Work out the finished part from the listing and answer in its coordinate system (mm). Face numbers are marked on the shaded views. Give positions to 0.01 mm unless a question says otherwise; leave off trailing zeros. Order: outer loops, then holes, each group sorted by start corner. A loop starts at its lowest first (then second) coordinate and runs counter-clockwise, first axis right, second up. Notation, with made-up numbers: M 36.25,50.5 L 42.25,50.5 A12 cw 42.25,64.5 Z; hole C 31,58 d1. An arc over 180 degrees is marked long. One line per item, written item: value.
from build123d import *

# Parameters (mm, degrees)
F1_DEPTH = 4
F2_R     = 1.99999
F3_R     = 1


# Not quite as in the source:
# - a fillet or chamfer is up to 0.001 mm smaller than in the source, because OpenCascade refuses the exact size


with BuildPart() as f1:
    # F0 (on Top) → F1 (new body)
    with BuildSketch(Plane.XY):
        Polygon((-28, 2), (-33, 2), (-33, -2), (-28, -2), (-28, -5), (-25, -5), (-25, -2), (25, -2), (25, -5), (28, -5), (28, -2), (33, -2), (33, 2), (28, 2), (28, 5), (25, 5), (25, 2), (-25, 2), (-25, 5), (-28, 5), align=None)
    extrude(amount=F1_DEPTH)

    # F2 (radius 2 in the source; OpenCascade refuses exactly that, so slightly less here)
    f2_edges = [f1.edges().sort_by_distance(p)[0] for p in [
        (33, -2, 2),
        (33, 2, 2),
        (-33, -2, 2),
        (-33, 2, 2),
    ]]
    fillet(f2_edges, radius=F2_R)

    # F3
    f3_edges = [f1.edges().sort_by_distance(p)[0] for p in [
        (-28, -5, 2),
        (-28, 5, 2),
        (28, -5, 2),
        (28, 5, 2),
        (-25, -5, 2),
        (-25, 5, 2),
        (25, 5, 2),
        (25, -5, 2),
        (25, -2, 2),
        (25, 2, 2),
        (-25, 2, 2),
        (-25, -2, 2),
    ]]
    fillet(f3_edges, radius=F3_R)


solid = f1.part
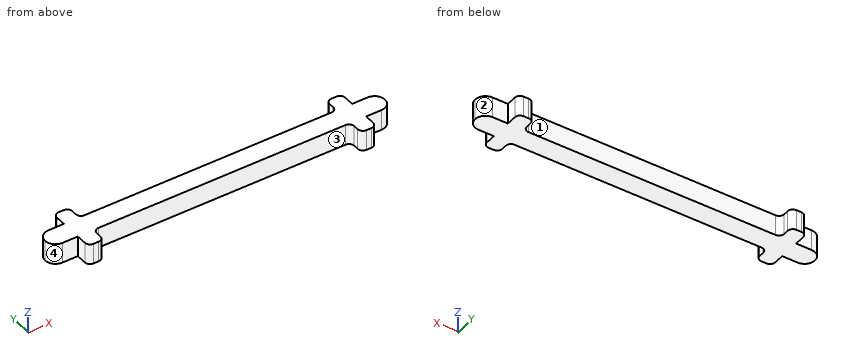
(1) Given P1, Ø0.6, axis at y = 3.5, z = 2.5, coming from the +X side; P2, Ø1.6, axis at y = -3, z = 2, coming from the -X side; P3, Ø2, axis at x = -10.5, z = 1.5, coming from the +Y side; P4, Ø6, axis at x = -6, y = 1, coming from the -Z side, each flat-ended and moving along its own axis, determine where each tip first touches the part or whether it passes through.
Findings:
P1: stops at x = 28
P2: stops at x = -28
P3: stops at y = 2
P4: stops at z = 0
(2) Determine the mould class of the marked faces 1, 2, 3 and 4 for opening direction X: pulls with the +X half, pulls with the -X half, needs draft (parallel to the pull), parting line crosses it, or undercut.
Findings:
face 1: undercut
face 2: pulls with the +X half
face 3: undercut
face 4: pulls with the -X half
(3) Find the intervals of material crossed by probe 1 along Y at (x, z) = (-13.5, 3.4); probe 2 along X at (y, z) = (4.25, 1.45); probe 3 along X at (y, z) = (-4.5, 0.6), in increasing order. Write a range as from..to.
Findings:
probe 1: y = -2..2
probe 2: x = -27.97..-25.03, 25.03..27.97
probe 3: x = -27.87..-25.13, 25.13..27.87
(4) Section A-A, the plane x = -2 is taken. Give the vertices of the cut face in (y, z), then the cut area to 3 significant figures.
Findings:
outline: M -2,0 L 2,0 L 2,4 L -2,4 Z
area: 16.0 mm^2
